Here's the drawing with two shaded views (mm, measured from the low corner). I have some questions. A direction names the side the tool comes from. Round coordinates to 2 decimals unless told otherwise and drop trailing zeros. Loops run counter-clockwise (first coordinate to the right, second up) from the corner with the lowest first, then second, coordinate; pieces in that order, holes last.
(1) Thinking about a two-plate mould opening in X: for the marked faces 3, 4, 5 and 6, which applies, released by +X, released by -X, zero draft, split by the parting line, or undercut?
(2) If I drill on line 1 along X through (y, z) = (6.5, 13.5) (1 decimal); line 2 along Y through (x, z) = (23, 12.75); line 3 along Y through (x, z) = (8.5, 2.5), over which ranges is the centre line in solid material (lowest first)?
(3) I want a section at B-B on y = 11.25. Write out the boundary of the cut face in (x, z).
(4) Will these pins go through, and if not, where does the flat tip stop? pin 1 Ø13.5 at (x, z) = (21.5, 14.5) entering from +Y; pin 2 Ø1.5 at (y, z) = (13, 6) entering from +X; pin 3 Ø1.5 at (x, y) = (11.5, 13) entering from -Z; pin 4 Ø8 at (x, z) = (13, 18) entering from -Y (1 decimal).
(5) Which directions (+Z, -Z, +X, -X, +Y, -Y) give clear straight access to the entire face, cutting with the end or side of a thin tool? Please do the marked faces 1 and 2.
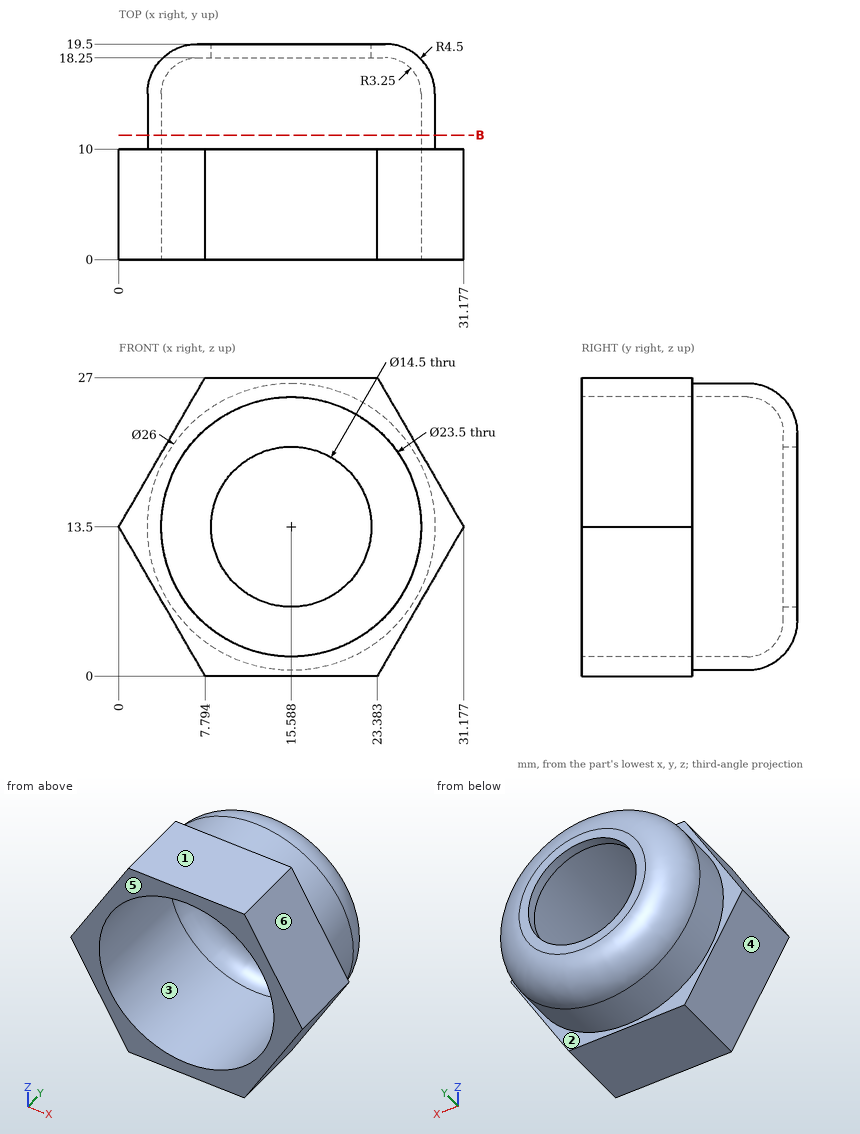
Filled sheet:
1. face 3: undercut
1. face 4: released by -X
1. face 5: zero draft
1. face 6: released by +X
2. line 1: x = 0 to 3.8, 27.3 to 31.2
2. line 2: y = 18.25 to 19.5
2. line 3: y = 0 to 10
3. outline: circle Ø26 at (15.59, 13.5); hole circle Ø23.5 at (15.59, 13.5)
4. pin 1: stops at y = 19.5
4. pin 2: stops at x = 26.7
4. pin 3: stops at z = 0.94
4. pin 4: stops at y = 18.2
5. face 1: +Z, +X, -X, +Y, -Y
5. face 2: +Y
